Part model, mm, in its own coordinate system. Face numbers are marked on the shaded views. A direction names the side the tool comes from. Give positions to 0.01 mm unless a question says otherwise; leave off trailing zeros. Order: outer loops, then holes, each group sorted by start corner. A loop starts at its lowest first (then second) coordinate and runs counter-clockwise, first axis right, second up. Notation, with made-up numbers: (18, 85.5) - (59, 85.5) arc R20 ccw to (59, 96.5) - close; hole circle Ø2 at (11.5, -14). An arc over 180 degrees is marked (long way). One line per item, written item: value.
```python
from build123d import *

# Parameters (mm, degrees)
SKETCH1_W           = 13
SKETCH1_H           = 13
BOSS_EXTRUDE1_DEPTH = 3
SKETCH2_R           = 6
CUT_EXTRUDE1_DEPTH  = 3
SKETCH4_W           = 3
SKETCH4_H           = 5
BOSS_EXTRUDE2_DEPTH = 3


with BuildPart() as part:
    # Sketch1 → Boss-Extrude1 (new body)
    with BuildSketch(Plane(origin=(0, 0, 0), x_dir=(1, 0, 0), z_dir=(0, 1, 0))):
        Rectangle(SKETCH1_W, SKETCH1_H)
    extrude(amount=BOSS_EXTRUDE1_DEPTH)

    # Sketch2 → Cut-Extrude1 (cut)
    with BuildSketch(Plane(origin=(0, 3, 0), x_dir=(1, 0, 0), z_dir=(0, 1, 0))):
        with Locations(Location((0, 0, 0), (0, 0, 270))):
            Circle(SKETCH2_R)
    extrude(amount=-CUT_EXTRUDE1_DEPTH, mode=Mode.SUBTRACT)

    # Sketch4 → Boss-Extrude2 (add)
    with BuildSketch(Plane(origin=(0, 3, 0), x_dir=(1, 0, 0), z_dir=(0, 1, 0))):
        with Locations((-8, 0)):
            Rectangle(SKETCH4_W, SKETCH4_H)
        with Locations((8, 0)):
            Rectangle(SKETCH4_W, SKETCH4_H)
    extrude(amount=-BOSS_EXTRUDE2_DEPTH)


solid = part.part
```
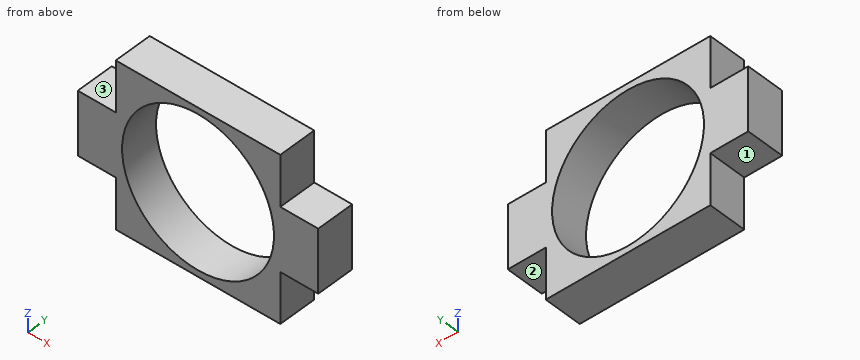
1) Pin check, flat tips, straight feed: pin 1 (1.5 mm diameter, centred on x = -8.5, y = 1.5, fed in from +Z); pin 2 (1.5 mm diameter, centred on y = 1, z = 3.5, fed in from +X); pin 3 (1.5 mm diameter, centred on x = 8.5, y = 1.5, fed in from -Z). Stop position of each tip, or through.
Outcome:
pin 1: stops at z = 2.5
pin 2: stops at x = 6.5
pin 3: stops at z = -2.5
2) Drill centre lines: line 1 along X through (y, z) = (2.3, 0); line 2 along Z through (x, y) = (-7, 1.2); line 3 along Z through (x, y) = (-3.75, 0.9). Where is each one in solid material? Low to high. Write a range as from..to.
Outcome:
line 1: x = -9.5..-6, 6..9.5
line 2: z = -2.5..2.5
line 3: z = -6.5..-4.68, 4.68..6.5
3) Which spindle directions (+Z, -Z, +X, -X, +Y, -Y) get a long thin tool onto all of the face, cutting with end or side? Do the marked faces 1, 2 and 3. Say none if no direction does.
Outcome:
face 1: -Z, -X, +Y, -Y
face 2: -Z, +X, +Y, -Y
face 3: +Z, -X, +Y, -Y
4) Cut at C-C, the plane x = 0. Give the cut face in (y, z), then the cut area to 3 significant figures.
Outcome:
outline: (0, -6.5) - (3, -6.5) - (3, -6) - (0, -6) - close; (0, 6) - (3, 6) - (3, 6.5) - (0, 6.5) - close
area: 3.00 mm^2
5) Cut at B-B, the plane z = 0. Give the cut face in (x, y), then the cut area to 3 significant figures.
Outcome:
outline: (-9.5, 0) - (-6, 0) - (-6, 3) - (-9.5, 3) - close; (6, 0) - (9.5, 0) - (9.5, 3) - (6, 3) - close
area: 21.0 mm^2
6) Cut at A-A, the plane y = 0.85. Give the cut face in (x, z).
Outcome:
outline: (-9.5, -2.5) - (-6.5, -2.5) - (-6.5, -6.5) - (6.5, -6.5) - (6.5, -2.5) - (9.5, -2.5) - (9.5, 2.5) - (6.5, 2.5) - (6.5, 6.5) - (-6.5, 6.5) - (-6.5, 2.5) - (-9.5, 2.5) - close; hole circle Ø12 at (0, 0)
